Design review of the part built by this model. Coordinates are the model's own, in mm. Face numbers are marked on the shaded views. A direction names the side the tool comes from. Coordinates: 2 decimals unless noted, no trailing zeros. Write each loop counter-clockwise with the first axis right and the second up, starting at its lowest first coordinate (ties: lowest second). Pieces come first, ordered by that corner, then holes. Notation, with made-up numbers: (40.25, -19) - (53.25, -19) arc R38 ccw to (53.25, 19) - close; hole circle Ø5 at (-11, 13). An arc over 180 degrees is marked (long way). One line per item, written item: value.
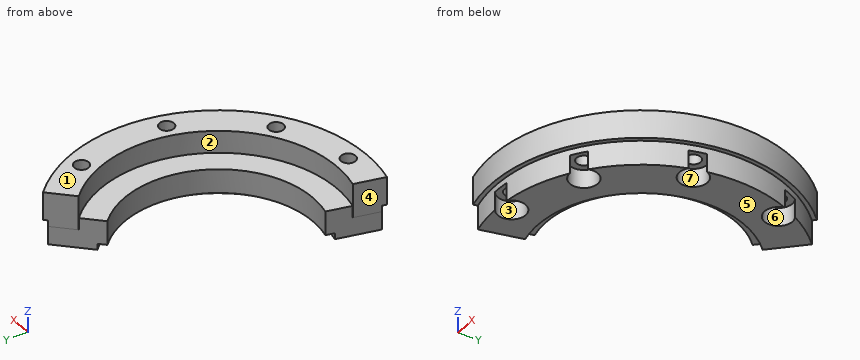
from build123d import *

# Parameters (mm, degrees)
BOSS_1_DEPTH  = 5.6
BOSS_2_DEPTH  = 4.95
CUT_3_DEPTH   = 1.1
CUT_4_DEPTH   = 1.1
S_HOLE5_R     = 1.2
HOLE_5_DEPTH  = 8.8
S_HOLE6_R     = 2.3
HOLE_6_DEPTH  = 3.1
S_HOLE7_R     = 1.2
HOLE_7_DEPTH  = 8.8
S_HOLE8_R     = 2.3
HOLE_8_DEPTH  = 3.1
S_HOLE9_R     = 1.2
HOLE_9_DEPTH  = 8.8
S_HOLE10_R    = 2.3
HOLE_10_DEPTH = 3.1
S_HOLE11_R    = 1.2
HOLE_11_DEPTH = 8.8
S_HOLE12_R    = 2.3
HOLE_12_DEPTH = 3.1


with BuildPart() as part:
    # S_prism1 → Boss_1 (new body)
    with BuildSketch(Plane.XY.offset(24.6)):
        with BuildLine():
            Line((-5.951278632, -23.869274866), (-4.741669154, -19.017796235))
            ThreePointArc((-4.741669154, -19.017796235), (17.05897164, -9.651501778), (13.859292911, 13.859292911))
            Line((13.859292911, 13.859292911), (17.394826817, 17.394826817))
            ThreePointArc((17.394826817, 17.394826817), (21.41075012, -12.113619579), (-5.951278632, -23.869274866))
        make_face()
    extrude(amount=BOSS_1_DEPTH)

    # S_prism2 → Boss_2 (add)
    with BuildSketch(Plane.XY.offset(21.6)):
        with BuildLine():
            Line((-5.753596984, -23.197114513), (-3.755485898, -15.14121282))
            ThreePointArc((-3.755485898, -15.14121282), (13.577548857, -7.681807538), (11.044334296, 11.017380812))
            Line((11.044334296, 11.017380812), (16.920486517, 16.879192399))
            ThreePointArc((16.920486517, 16.879192399), (20.801501133, -11.768923086), (-5.753596984, -23.197114513))
        make_face()
    extrude(amount=BOSS_2_DEPTH)

    # S_pcut3 → Cut_3 (cut)
    with BuildSketch(Plane.XY.offset(24.5)):
        with BuildLine():
            Line((-6.418712319, -23.954960492), (-6.185775178, -23.085627248))
            ThreePointArc((-6.185775178, -23.085627248), (20.801501133, -11.768923086), (16.602335054, 17.192221228))
            Line((16.602335054, 17.192221228), (17.227527587, 17.839627048))
            ThreePointArc((17.227527587, 17.839627048), (21.584821259, -12.212104291), (-6.418712319, -23.954960492))
        make_face()
    extrude(amount=CUT_3_DEPTH, mode=Mode.SUBTRACT)

    # S_pcut4 → Cut_4 (cut)
    with BuildSketch(Plane.XY.offset(21.5)):
        with BuildLine():
            Line((-4.399923767, -16.420739047), (-4.011695199, -14.971850307))
            ThreePointArc((-4.011695199, -14.971850307), (13.490513287, -7.632565182), (10.767204742, 11.149766905))
            Line((10.767204742, 11.149766905), (11.809192298, 12.228776606))
            ThreePointArc((11.809192298, 12.228776606), (14.796046831, -8.371200522), (-4.399923767, -16.420739047))
        make_face()
    extrude(amount=CUT_4_DEPTH, mode=Mode.SUBTRACT)

    # S_hole5 → Hole_5 (cut)
    with BuildSketch(Plane.XY.offset(21.5)):
        with Locations(Location((19.938771315, 9.297601758, 0), (0, 0, 180))):
            Circle(S_HOLE5_R)
    extrude(amount=HOLE_5_DEPTH, mode=Mode.SUBTRACT)

    # S_hole6 → Hole_6 (cut)
    with BuildSketch(Plane.XY.offset(21.5)):
        with Locations((19.938771315, 9.297601758)):
            Circle(S_HOLE6_R)
    extrude(amount=HOLE_6_DEPTH, mode=Mode.SUBTRACT)

    # S_hole7 → Hole_7 (cut)
    with BuildSketch(Plane.XY.offset(21.5)):
        with Locations(Location((21.250368178, -5.694018992, 0), (0, 0, 180))):
            Circle(S_HOLE7_R)
    extrude(amount=HOLE_7_DEPTH, mode=Mode.SUBTRACT)

    # S_hole8 → Hole_8 (cut)
    with BuildSketch(Plane.XY.offset(21.5)):
        with Locations((21.250368178, -5.694018992)):
            Circle(S_HOLE8_R)
    extrude(amount=HOLE_8_DEPTH, mode=Mode.SUBTRACT)

    # S_hole9 → Hole_9 (cut)
    with BuildSketch(Plane.XY.offset(21.5)):
        with Locations(Location((12.6186816, -18.021344974, 0), (0, 0, 180))):
            Circle(S_HOLE9_R)
    extrude(amount=HOLE_9_DEPTH, mode=Mode.SUBTRACT)

    # S_hole10 → Hole_10 (cut)
    with BuildSketch(Plane.XY.offset(21.5)):
        with Locations((12.6186816, -18.021344974)):
            Circle(S_HOLE10_R)
    extrude(amount=HOLE_10_DEPTH, mode=Mode.SUBTRACT)

    # S_hole11 → Hole_11 (cut)
    with BuildSketch(Plane.XY.offset(21.5)):
        with Locations(Location((0.767788927, -21.986598194, 0), (0, 0, 180))):
            Circle(S_HOLE11_R)
    extrude(amount=HOLE_11_DEPTH, mode=Mode.SUBTRACT)

    # S_hole12 → Hole_12 (cut)
    with BuildSketch(Plane.XY.offset(21.5)):
        with Locations((0.767788927, -21.986598194)):
            Circle(S_HOLE12_R)
    extrude(amount=HOLE_12_DEPTH, mode=Mode.SUBTRACT)


solid = part.part
1. Consider section B-B, the plane z = 27.75. Write out the cut boundary in (x, y).
Answer block:
outline: (-5.95, -23.87) arc R24.6 ccw to (17.39, 17.39) - (13.86, 13.86) arc R19.6 cw to (-4.74, -19.02) - close; hole circle Ø2.4 at (0.77, -21.99); hole circle Ø2.4 at (12.62, -18.02); hole circle Ø2.4 at (19.94, 9.3); hole circle Ø2.4 at (21.25, -5.69)
2. Wall thickness on line 1 along Y through (x, z) = (12.5, 27); line 2 along X through (y, z) = (-18.5, 24.25); line 3 along Y through (x, z) = (20, 25): over which ranges is each line inside the solid? List them lowest first.
Answer block:
line 1: y = -21.19 to -19.22, -16.83 to -15.1
line 2: x = -4.59 to 10.37, 14.87 to 15.13
line 3: y = -13.08 to 8.1, 10.5 to 13.08
3. Consider section A-A, the plane y = -14. Write out the cut boundary in (x, z).
Answer block:
outline: (6.88, 22.6) - (9.64, 22.6) - (9.64, 21.6) - (19.37, 21.6) - (19.37, 25.6) - (20.23, 25.6) - (20.23, 30.2) - (13.72, 30.2) - (13.72, 26.55) - (6.88, 26.55) - close
4. For the marked faces 1, 2 and 3, list the 3-axis set-ups (+Z, -Z, +X, -X, +Y, -Y) from which the entire face can be reached by the end or side of a thin tool; tool diameter is ignored.
Answer block:
face 1: +Z, +X, -X, +Y, -Y
face 2: +Z
face 3: -Z
5. Mouldability with a two-part tool opening along Y and no side actions: class the marked faces 4, 5, 6 and 7 as released by +Y, released by -Y, zero draft, split by the parting line, or undercut.
Answer block:
face 4: released by +Y
face 5: zero draft
face 6: undercut
face 7: undercut
6. Consider section C-C, the plane x = 7. Write out the cut boundary in (y, z), then the cut area to 3 significant figures.
Answer block:
outline: (-23.58, 25.6) - (-22.85, 25.6) - (-22.85, 21.6) - (-15.49, 21.6) - (-15.49, 22.6) - (-13.94, 22.6) - (-13.94, 26.55) - (-18.31, 26.55) - (-18.31, 30.2) - (-23.58, 30.2) - close
area: 62.5 mm^2
7. Consider section D-D, the plane z = 23.5. Write out the cut boundary in (x, y).
Answer block:
outline: (-5.75, -23.2) arc R23.9 ccw to (-0.52, -23.89) arc R2.3 cw (long way) to (2.18, -23.8) arc R23.9 ccw to (12.58, -20.32) arc R2.3 cw (long way) to (14.79, -18.77) arc R23.9 ccw to (22.7, -7.48) arc R2.3 cw (long way) to (23.4, -4.87) arc R23.9 ccw to (22.2, 8.86) arc R2.3 cw (long way) to (21.06, 11.31) arc R23.9 ccw to (16.92, 16.88) - (11.04, 11.02) arc R15.6 cw to (-3.76, -15.14) - close
8. Insertion check: pin 1 Ø1.3 at (x, y) = (20.5, -5) entering from -Z; pin 2 Ø2 at (x, z) = (3, 22.5) entering from -Y; pin 3 Ø1.5 at (y, z) = (-17, 25.5) entering from +X. Each pin has a flat end and moves straight along its axis. Give the tip position at first contact, or say it passes through.
Answer block:
pin 1: stops at z = 24.6
pin 2: stops at y = -23.8
pin 3: stops at x = 18.46
